Input: part model. Units: mm. Frame: model coordinates. A direction names the side the tool comes from. Coordinates: 2 decimals unless noted, no trailing zeros. Write each loop counter-clockwise with the first axis right and the second up, starting at its lowest first coordinate (ties: lowest second). Pieces come first, ordered by that corner, then holes. Notation, with made-up numbers: (88.25, -19.75) - (107.25, -19.75) arc R16 cw to (107.25, 11.25) - close; hole circle Ø4 at (4, -1). An arc over 180 degrees is marked (long way). Use a Markdown table: item, result. Add a question column.
Q1. Pin query (flat end, axial travel): P1, Ø0.9, axis at x = 0, y = 3, coming from the +Z side (3 decimals); P2, Ø3.5, axis at x = 0, z = 10.5, coming from the +Y side; P3, Ø1.9, axis at y = 0.5, z = 1.5, coming from the -X side. Return the tip coordinate at first contact, or that it passes through.
Q2. Material intervals for probe 1 along Y at (x, z) = (0, -8); probe 2 along X at (y, z) = (0, 9.5); probe 3 along Y at (x, z) = (0, -11.5), sorted ascending. Write a range as from..to.
Q3. Section query C-C (z = 0). Return the cut outline in (x, y).
Q4. Set-up query: faces 1 (the face through (-2.34, 1, 1)), 2 (the face through (-1.5, 0.07, -9.13)), 3 (the face through (0, -2, -11)). Return all of +Z, -Z, +X, -X, +Y, -Y with unobstructed straight access to the full face (end or side cutting, diameter ignored); none if empty.
Q5. Section query B-B (x = 2.75). Return the cut outline in (y, z) (3 decimals).
Q6. Section query A-A (z = 12.25). Return the cut outline in (x, y), then the cut area to 3 significant figures.
Q7. Mould query, pull axis Z, two halves, no side actions, for faces 4 (the face through (1.5, 0.07, 9.13)), 5 (the face through (0, 2.5, -3.865)), 6 (the face through (0.29, -1.22, -0.27)). Classes: released by +Z, released by -Z, zero draft, split by the parting line, or undercut.
Q8. Section query D-D (z = 6.5). Return the cut outline in (x, y).
from build123d import *

# Parameters (mm, degrees)
BOSS_EXTRUDE1_DEPTH                                 = 13.865
BOSS_EXTRUDE1_DEPTH_BACK                            = 13.865
SKETCH1_R                                           = 3
CUT_EXTRUDE1_DEPTH                                  = 5
CUT_EXTRUDE2_DEPTH                                  = 5
CUT_EXTRUDE5_DEPTH                                  = 5
CUT_EXTRUDE6_START                                  = -5
CUT_EXTRUDE6_DEPTH                                  = 5
CSK_FOR_M3_COUNTERSUNK_FLAT_HEAD_SCREW1_D           = 3
CSK_FOR_M3_COUNTERSUNK_FLAT_HEAD_SCREW1_DEPTH       = 9.098709071
CSK_FOR_M3_COUNTERSUNK_FLAT_HEAD_SCREW1_CSINK_D     = 3.5
CSK_FOR_M3_COUNTERSUNK_FLAT_HEAD_SCREW1_CSINK_ANGLE = 90
CSK_FOR_M3_COUNTERSUNK_FLAT_HEAD_SCREW1_TIP         = 0.901290929
CSK_FOR_M3_COUNTERSUNK_FLAT_HEAD_SCREW2_D           = 3
CSK_FOR_M3_COUNTERSUNK_FLAT_HEAD_SCREW2_DEPTH       = 9.098709071
CSK_FOR_M3_COUNTERSUNK_FLAT_HEAD_SCREW2_CSINK_D     = 3.5
CSK_FOR_M3_COUNTERSUNK_FLAT_HEAD_SCREW2_CSINK_ANGLE = 90
CSK_FOR_M3_COUNTERSUNK_FLAT_HEAD_SCREW2_TIP         = 0.901290929
SKETCH14_W                                          = 7.4
SKETCH14_H                                          = 4
CUT_EXTRUDE9_DEPTH                                  = 3
SKETCH15_R                                          = 1.25
CUT_EXTRUDE10_DEPTH                                 = 16.157632566


with BuildPart() as part:
    # Sketch1 → Boss-Extrude1 (new, two sides: drawn at the far end of the back side and taken through both)
    with BuildSketch(Plane.XY.offset(-BOSS_EXTRUDE1_DEPTH_BACK)):
        Circle(SKETCH1_R)
    extrude(amount=BOSS_EXTRUDE1_DEPTH + BOSS_EXTRUDE1_DEPTH_BACK)

    # Sketch2 → Cut-Extrude1 (cut)
    with BuildSketch(Plane.XY.offset(13.865)):
        with BuildLine():
            Line((-2.236067977, 2), (2.236067977, 2))
            ThreePointArc((2.236067977, 2), (0, 3), (-2.236067977, 2))
        make_face()
        with BuildLine():
            Line((-2.236067977, -2), (2.236067977, -2))
            ThreePointArc((2.236067977, -2), (0, -3), (-2.236067977, -2))
        make_face()
    extrude(amount=-CUT_EXTRUDE1_DEPTH, mode=Mode.SUBTRACT)

    # Sketch3 → Cut-Extrude2 (cut)
    with BuildSketch(Plane(origin=(0, 0, -13.865), x_dir=(-1, 0, 0), z_dir=(0, 0, -1))):
        with BuildLine():
            Line((-2.236067977, 2), (2.236067977, 2))
            ThreePointArc((2.236067977, 2), (0, 3), (-2.236067977, 2))
        make_face()
        with BuildLine():
            Line((-2.236067977, -2), (2.236067977, -2))
            ThreePointArc((2.236067977, -2), (0, -3), (-2.236067977, -2))
        make_face()
    extrude(amount=-CUT_EXTRUDE2_DEPTH, mode=Mode.SUBTRACT)

    # Sketch4 → Cut-Extrude5 (cut)
    with BuildSketch(Plane(origin=(0, 0, -8.865), x_dir=(-1, 0, 0), z_dir=(0, 0, -1))):
        with BuildLine():
            Line((-2.1, 2.142428529), (2.1, 2.142428529))
            ThreePointArc((2.1, 2.142428529), (0, 3), (-2.1, 2.142428529))
        make_face()
    extrude(amount=-CUT_EXTRUDE5_DEPTH, mode=Mode.SUBTRACT)

    # Sketch5 → Cut-Extrude6 (cut)
    with BuildSketch(Plane.XY.offset(8.865).offset(CUT_EXTRUDE6_START)):
        with BuildLine():
            Line((-2.1, 2.142428529), (2.1, 2.142428529))
            ThreePointArc((2.1, 2.142428529), (0, 3), (-2.1, 2.142428529))
        make_face()
    extrude(amount=CUT_EXTRUDE6_DEPTH, mode=Mode.SUBTRACT)

    # CSK for M3 Countersunk Flat Head Screw1
    with Locations(Plane(origin=(0, 0, -13.865), x_dir=(-1, 0, 0), z_dir=(0, 0, -1))):
        with Locations((0, 0)):
            CounterSinkHole(CSK_FOR_M3_COUNTERSUNK_FLAT_HEAD_SCREW1_D / 2, CSK_FOR_M3_COUNTERSUNK_FLAT_HEAD_SCREW1_CSINK_D / 2, depth=CSK_FOR_M3_COUNTERSUNK_FLAT_HEAD_SCREW1_DEPTH, counter_sink_angle=CSK_FOR_M3_COUNTERSUNK_FLAT_HEAD_SCREW1_CSINK_ANGLE)
            with Locations((0, 0, -(CSK_FOR_M3_COUNTERSUNK_FLAT_HEAD_SCREW1_DEPTH + CSK_FOR_M3_COUNTERSUNK_FLAT_HEAD_SCREW1_TIP / 2))):  # 118° drill point
                Cone(0, CSK_FOR_M3_COUNTERSUNK_FLAT_HEAD_SCREW1_D / 2, CSK_FOR_M3_COUNTERSUNK_FLAT_HEAD_SCREW1_TIP, mode=Mode.SUBTRACT)

    # CSK for M3 Countersunk Flat Head Screw2
    with Locations(Plane.XY.offset(13.865)):
        with Locations((0, 0)):
            CounterSinkHole(CSK_FOR_M3_COUNTERSUNK_FLAT_HEAD_SCREW2_D / 2, CSK_FOR_M3_COUNTERSUNK_FLAT_HEAD_SCREW2_CSINK_D / 2, depth=CSK_FOR_M3_COUNTERSUNK_FLAT_HEAD_SCREW2_DEPTH, counter_sink_angle=CSK_FOR_M3_COUNTERSUNK_FLAT_HEAD_SCREW2_CSINK_ANGLE)
            with Locations((0, 0, -(CSK_FOR_M3_COUNTERSUNK_FLAT_HEAD_SCREW2_DEPTH + CSK_FOR_M3_COUNTERSUNK_FLAT_HEAD_SCREW2_TIP / 2))):  # 118° drill point
                Cone(0, CSK_FOR_M3_COUNTERSUNK_FLAT_HEAD_SCREW2_D / 2, CSK_FOR_M3_COUNTERSUNK_FLAT_HEAD_SCREW2_TIP, mode=Mode.SUBTRACT)

    # Sketch14 → Cut-Extrude9 (cut)
    with BuildSketch(Plane(origin=(-5.34, 0, 0), x_dir=(0, 0, -1), z_dir=(1, 0, 0))):
        Rectangle(SKETCH14_W, SKETCH14_H)
    extrude(amount=CUT_EXTRUDE9_DEPTH, mode=Mode.SUBTRACT)

    # Sketch15 → Cut-Extrude10 (cut, through all)
    with BuildSketch(Plane.ZY.offset(2.34)):
        Circle(SKETCH15_R)
    extrude(amount=-CUT_EXTRUDE10_DEPTH, mode=Mode.SUBTRACT)


solid = part.part
Values follow:
| question | item | result |
|---|---|---|
| 1 | P1 | z = 3.865 |
| 1 | P2 | y = 2.14 |
| 1 | P3 | x = -2.34 |
| 2 | probe 1 | -3..-1.5, 1.5..2.14 |
| 2 | probe 2 | -3..-1.5, 1.5..3 |
| 2 | probe 3 | -2..-1.5, 1.5..2 |
| 3 | outline | (-2.34, -1.88) arc R3 ccw to (2.73, -1.25) - (-2.34, -1.25) - close; (-2.34, 1.25) - (2.73, 1.25) arc R3 ccw to (-2.34, 1.88) - close |
| 4 | face 1 | -X, +Y, -Y |
| 4 | face 2 | -Z |
| 4 | face 3 | -Z, +X, -X, -Y |
| 5 | outline | (-1.199, -13.865) - (1.199, -13.865) - (1.199, -0.354) arc R1.25 cw to (-1.199, -0.354) - close; (-1.199, 0.354) arc R1.25 cw to (1.199, 0.354) - (1.199, 13.865) - (-1.199, 13.865) - close |
| 6 | outline | (-2.24, -2) - (2.24, -2) arc R3 ccw to (2.24, 2) - (-2.24, 2) arc R3 ccw to start; hole circle Ø3 at (0, 0) |
| 6 | area | 15.0 mm2 |
| 7 | face 4 | zero draft |
| 7 | face 5 | released by -Z |
| 7 | face 6 | undercut |
| 8 | outline | (-2.1, 2.14) arc R3 ccw (long way) to (2.1, 2.14) - close; hole circle Ø3 at (0, 0) |
